```python
from build123d import *

# Parameters (mm, degrees)
SKETCH1_R           = 4
BOSS_EXTRUDE1_DEPTH = 560
SKETCH2_R           = 17
BOSS_EXTRUDE2_DEPTH = 250


with BuildPart() as part:
    # Sketch1 → Boss-Extrude1 (new body)
    with BuildSketch(Plane.XY):
        Circle(SKETCH1_R)
    extrude(amount=BOSS_EXTRUDE1_DEPTH)

    # Sketch2 → Boss-Extrude2 (add, symmetric)
    with BuildSketch(Plane.XY.offset(280)):
        Circle(SKETCH2_R)
    extrude(amount=BOSS_EXTRUDE2_DEPTH, both=True)


solid = part.part
```
CAD build for the part. Positions are in the model's coordinates, mm. Give positions to 0.01 mm unless a question says otherwise; leave off trailing zeros. Order: outer loops, then holes, each group sorted by start corner. A loop starts at its lowest first (then second) coordinate and runs counter-clockwise, first axis right, second up. Notation, with made-up numbers: M -13.5,-39 L -0.5,-39 A27 cw -0.5,-15 Z; hole C 59,29.5 d4. An arc over 180 degrees is marked long. Put each result on its own line as item: value. Start each with the question number.
(1) Drill centre lines: line 1 along Z through (x, y) = (-14.5, -4); line 2 along Y through (x, z) = (-1, 398.5). Where is each one in solid material? Low to high.
(2) Saw through at C-C, the plane x = 10. Write the cut outline in (y, z), then the cut area to 3 significant figures.
(3) Flat gauge pins, fed straight in: pin 1 Ø5 at (x, z) = (8, 114.5) entering from -Y; pin 2 Ø5 at (x, y) = (4.5, -6) entering from -Z; pin 3 Ø5 at (y, z) = (-9.5, 201.5) entering from +X. Where does each tip first touch, or does it go through?
(4) Saw through at B-B, the plane y = 9. Write the cut outline in (x, z).
(5) Saw through at A-A, the plane z = 91. Write the cut outline in (x, y), then the cut area to 3 significant figures.
Check result:
1. line 1: z = 30 to 530
1. line 2: y = -16.97 to 16.97
2. outline: M -13.75,30 L 13.75,30 L 13.75,530 L -13.75,530 Z
2. area: 13,700 mm2
3. pin 1: stops at y = -16.09
3. pin 2: stops at z = 30
3. pin 3: stops at x = 15.49
4. outline: M -14.42,30 L 14.42,30 L 14.42,530 L -14.42,530 Z
5. outline: C 0,0 d34
5. area: 908 mm2
